Drawing for the job (mm, zero at the part's lowest x, y, z). Coordinates: 2 decimals unless noted, no trailing zeros. Write each loop counter-clockwise with the first axis right and the second up, starting at its lowest first coordinate (ties: lowest second). Pieces come first, ordered by that corner, then holes. Notation, with made-up numbers: M -21.75,36 L 10.25,36 A14 cw 10.25,58 Z; hole C 66.25,-40 d11. An arc over 180 degrees is marked long. Use a Markdown table: item, result. Add a question column.
Q1. Slice it at B-B on y = 54.5. Write the cut outline in (x, z).
Q2. Pin check, flat tips, straight feed: pin 1 Ø5.5 at (x, z) = (108.5, 10.5) entering from -Y; pin 2 Ø4 at (y, z) = (92.5, 14) entering from +X; pin 3 Ø6.5 at (y, z) = (97, 10.5) entering from -X. Stop position of each tip, or through.
Q3. Slice it at D-D on z = 2.25. Write the cut outline in (x, y) (1 decimal), then the cut area to 3 significant figures.
Q4. Wall check: L1, parallel to X at y = 5, z = 10.5; L2, parallel to Y at x = 89, z = 12; L3, parallel to Z at x = 127.5, y = 15. Give the ranges that are in metal, low to high. Write a range as from..to.
Q5. Slice it at A-A on z = 14.5. Write the cut outline in (x, y), then the cut area to 3 significant figures.
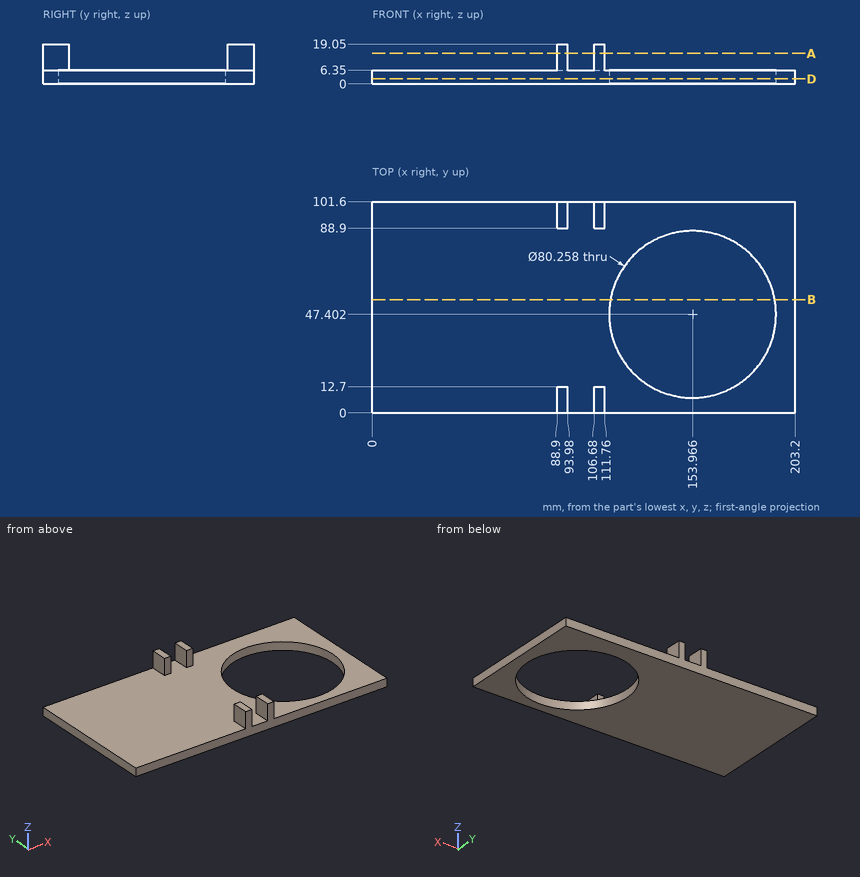
Recorded:
| question | item | result |
|---|---|---|
| 1 | outline | M 0,0 L 114.47,0 L 114.47,6.35 L 0,6.35 Z; M 193.46,0 L 203.2,0 L 203.2,6.35 L 193.46,6.35 Z |
| 2 | pin 1 | y = 0 |
| 2 | pin 2 | x = 111.76 |
| 2 | pin 3 | x = 88.9 |
| 3 | outline | M 0,0 L 203.2,0 L 203.2,101.6 L 0,101.6 Z; hole C 154,47.4 d80.3 |
| 3 | area | 15,600 mm² |
| 4 | L1 | 88.9..93.98, 106.68..111.76 |
| 4 | L2 | 0..12.7, 88.9..101.6 |
| 4 | L3 | 0..6.35 |
| 5 | outline | M 88.9,0 L 93.98,0 L 93.98,12.7 L 88.9,12.7 Z; M 88.9,88.9 L 93.98,88.9 L 93.98,101.6 L 88.9,101.6 Z; M 106.68,0 L 111.76,0 L 111.76,12.7 L 106.68,12.7 Z; M 106.68,88.9 L 111.76,88.9 L 111.76,101.6 L 106.68,101.6 Z |
| 5 | area | 258 mm² |
